Solid Edge part; units mm, degrees
sketch "Sketch1" plane through (0, 0, 0) normal (0, 0, 1) x (1, 0, 0)
  line L0 (-16, 34) -> (16, 34)
  line L1 (16, 34) -> (16, -34)
  line L2 (16, -34) -> (-16, -34)
  line L3 (-16, -34) -> (-16, 34)
  line L4 (-3, 27.5) -> (3, 27.5)
  line L5 (-3, 30.5) -> (3, 30.5)
  arc A0 (3, 30.5) -> (3, 27.5) centre (3, 29) cw
  arc A1 (-3, 27.5) -> (-3, 30.5) centre (-3, 29) cw
  arc A2 (3, -30.5) -> (3, -27.5) centre (3, -29) ccw
  line L6 (-3, -27.5) -> (3, -27.5)
  arc A3 (-3, -27.5) -> (-3, -30.5) centre (-3, -29) ccw
  line L7 (-3, -30.5) -> (3, -30.5)
  line L8 (-12, 20) -> (12, 20)
  line L9 (12, -20) -> (12, 20)
  line L10 (12, -20) -> (-12, -20)
  line L11 (-12, 20) -> (-12, -20)
extrude "Protrusion1" add sketch "Sketch1" along normal blind 4
sketch "Sketch2" plane through (0, 0, 0) normal (0, 0, 1) x (1, 0, 0)
  line L0 (4.5, 24) -> (-4.5, 24)
  line L1 (-4.5, 24) -> (-4.5, 20)
  line L2 (-4.5, 20) -> (4.5, 20)
  line L3 (4.5, 20) -> (4.5, 24)
extrude "ExtrudedCutout_3" cut sketch "Sketch2" along normal blind 2.5
fillet "Round_2" radius 2.5 4 edges at (16, 34, 2) (-16, 34, 2) (-16, -34, 2) (16, -34, 2)
sketch "Sketch3" plane through (0, 0, 0) normal (0, 0, 1) x (1, 0, 0)
  line L0 (4.5, -24) -> (-4.5, -24)
  line L1 (-4.5, -24) -> (-4.5, -20)
  line L2 (-4.5, -20) -> (4.5, -20)
  line L3 (4.5, -20) -> (4.5, -24)
extrude "Cutout1" cut sketch "Sketch3" along normal up to vertex (2.5 mm away)
sketch "Sketch4" plane through (0, 0, 0) normal (0, 0, -1) x (-1, 0, 0)
  line L0 (4.5, 22) -> (12, 22)
  line L1 (12, 22) -> (12, 20)
  line L2 (12, 20) -> (4.5, 20)
  line L3 (4.5, 20) -> (4.5, 22)
  line L4 (-12, 22) -> (-4.5, 22)
  line L5 (-4.5, 22) -> (-4.5, 20)
  line L6 (-4.5, 20) -> (-12, 20)
  line L7 (-12, 20) -> (-12, 22)
  line L8 (12, -22) -> (4.5, -22)
  line L9 (4.5, -22) -> (4.5, -20)
  line L10 (4.5, -20) -> (12, -20)
  line L11 (12, -20) -> (12, -22)
  line L12 (-12, -20) -> (-4.5, -20)
  line L13 (-4.5, -20) -> (-4.5, -22)
  line L14 (-4.5, -22) -> (-12, -22)
  line L15 (-12, -22) -> (-12, -20)
extrude "Cutout2" cut sketch "Sketch4" against normal up to vertex (2.5 mm away)
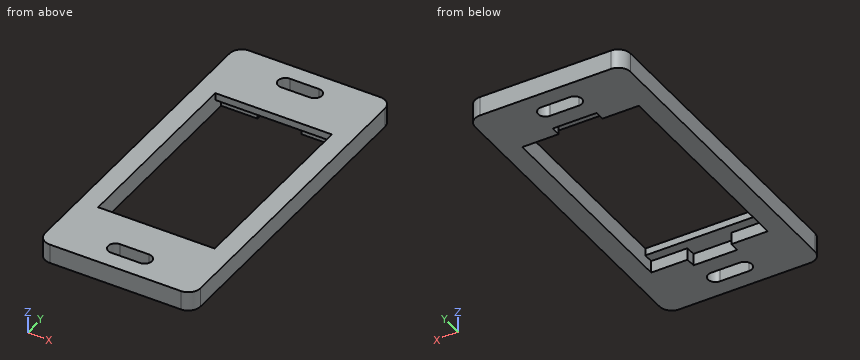
Source: CAD feature listing. Evaluate the final solid. Frame: model axes, mm. Coordinates: 2 decimals unless noted, no trailing zeros. Loops run counter-clockwise (first coordinate to the right, second up) from the corner with the lowest first, then second, coordinate; pieces in that order, holes last. Notation, with made-up numbers: M 74.5,35 L 84.5,35 A33 ccw 84.5,74 Z; hole C 80,66.5 d5. An arc over 180 degrees is marked long. Put each result on its own line as item: value. Start each with the question number.
1) Cut plane B-B on z = 1.2. Return the cut outline in (x, y), then the cut area to 3 significant figures.
2) Cut plane D-D on x = 9. Return the cut outline in (y, z), then the cut area to 3 significant figures.
3) Cut plane C-C on x = -1.5. Return the cut outline in (y, z), then the cut area to 3 significant figures.
4) Cut plane A-A on y = 29. Return the cut outline in (x, z).
5) Ray query, L1, parallel to Y at x = -0.5, z = 3.2; L2, parallel to Y at x = -3, z = 0.8; L3, parallel to Y at x = -9, z = 3.4. Return the intervals inside material, ascending. Write a range as from..to.
The answers:
1. outline: M -16,-31.5 A2.5 ccw -13.5,-34 L 13.5,-34 A2.5 ccw 16,-31.5 L 16,31.5 A2.5 ccw 13.5,34 L -13.5,34 A2.5 ccw -16,31.5 Z; hole M -12,-22 L -4.5,-22 L -4.5,-24 L 4.5,-24 L 4.5,-22 L 12,-22 L 12,22 L 4.5,22 L 4.5,24 L -4.5,24 L -4.5,22 L -12,22 Z; hole M -3,-30.5 L 3,-30.5 A1.5 ccw 3,-27.5 L -3,-27.5 A1.5 ccw Z; hole M -3,27.5 L 3,27.5 A1.5 ccw 3,30.5 L -3,30.5 A1.5 ccw Z
1. area: 1,030 mm²
2. outline: M -34,0 L -22,0 L -22,2.5 L -20,2.5 L -20,4 L -34,4 Z; M 20,2.5 L 22,2.5 L 22,0 L 34,0 L 34,4 L 20,4 Z
2. area: 102 mm²
3. outline: M -34,0 L -30.5,0 L -30.5,4 L -34,4 Z; M -27.5,0 L -24,0 L -24,2.5 L -20,2.5 L -20,4 L -27.5,4 Z; M 20,2.5 L 24,2.5 L 24,0 L 27.5,0 L 27.5,4 L 20,4 Z; M 30.5,0 L 34,0 L 34,4 L 30.5,4 Z
3. area: 68.0 mm²
4. outline: M -16,0 L -4.5,0 L -4.5,4 L -16,4 Z; M 4.5,0 L 16,0 L 16,4 L 4.5,4 Z
5. L1: y = -34..-30.5, -27.5..-20, 20..27.5, 30.5..34
5. L2: y = -34..-30.5, -27.5..-24, 24..27.5, 30.5..34
5. L3: y = -34..-20, 20..34
